```python
from build123d import *

# Parameters (mm, degrees)
F0_W        = 104.8084236681
F0_H        = 91.941319406
F1_DEPTH    = 3
F2_W        = 41.4473675191
F2_H        = 39.6052636206
F3_DEPTH    = 30
F4_T        = 3
F4_T3_DEPTH = 47.4473675191
F4_T5_DEPTH = 45.6052636206


# Not quite as in the source:
# - a shell that OpenCascade refuses in one call is made with other operations: the cavity is built on its own and cut out


with BuildPart() as f1:
    # F0 (on Top) → F1 (new body)
    with BuildSketch(Plane.XY):
        with Locations((0.5848687142, -2.3394748569)):
            Rectangle(F0_W, F0_H)
    extrude(amount=F1_DEPTH)

    # F2 (on face) → F3 (join)
    with BuildSketch(Plane.XY.offset(3)):
        with Locations((-0.575657934, -1.7269738019)):
            Rectangle(F2_W, F2_H)
    extrude(amount=F3_DEPTH)

    # F4: shell of thickness 3, made by hand


with BuildPart() as f4_core1:
    # F4_t2: copy of F1
    add(f1.part)

    # the walls: a layer under each face that stays
    f4_faces = [f4_core1.faces().sort_by_distance(p)[0] for p in [
        (0.5848687142, 43.6311848462, 1.5),
        (52.9890805483, -2.3394748569, 1.5),
        (-51.8193431199, -2.3394748569, 1.5),
        (-34.3512725085, -32.9865813255, 3),
        (0.5848687142, -48.3101345599, 1.5),
        (-0.575657934, 18.0756580085, 18),
        (-21.2993416935, -1.7269738019, 18),
        (-0.575657934, -21.5296056122, 18),
        (20.1480258256, -1.7269738019, 18),
        (-0.575657934, -1.7269738019, 33),
    ]]
    thicken(f4_faces, amount=-F4_T, mode=Mode.SUBTRACT)

    # F4_s4 → F4_t3 (cut)
    with BuildSketch(Plane.YZ.offset(-24.2993416935)):
        Polygon((18.1056580085, 3.03), (18.0756580085, 0), (15.0756580085, 0), (15.0756580085, 3), align=None)
        Polygon((-21.5596056122, 3.03), (-21.5296056122, 0), (-18.5296056122, 0), (-18.5296056122, 3), align=None)
    extrude(amount=F4_T3_DEPTH, mode=Mode.SUBTRACT)

    # F4_s6 → F4_t5 (cut)
    with BuildSketch(Plane.XZ.offset(-21.0756580085)):
        Polygon((-21.3293416935, 3.03), (-21.2993416935, 0), (-18.2993416935, 0), (-18.2993416935, 3), align=None)
        Polygon((20.1780258256, 3.03), (20.1480258256, 0), (17.1480258256, 0), (17.1480258256, 3), align=None)
    extrude(amount=F4_T5_DEPTH, mode=Mode.SUBTRACT)


with BuildPart() as f1_1:
    add(f1.part)

    # what is left inside the walls is the cavity
    f4_cavity = [f4_core1.part.solids().sort_by_distance(p)[0] for p in [
        (-0.575658, -7.327851, 0.03),
    ]]
    add(f4_cavity, mode=Mode.SUBTRACT)


solid = f1_1.part
```
Read the model definition and answer for the solid it produces. Units are mm, in the model's axes. A direction names the side the tool comes from. Coordinates: 2 decimals unless noted, no trailing zeros. Loops run counter-clockwise (first coordinate to the right, second up) from the corner with the lowest first, then second, coordinate; pieces in that order, holes last.
(1) The part is cut by section A-A (z = 14). Determine the outline of the cut face in (x, y).
Solution:
outline: (-21.3, -21.53) - (20.15, -21.53) - (20.15, 18.08) - (-21.3, 18.08) - close; hole (-18.3, -18.53) - (17.15, -18.53) - (17.15, 15.08) - (-18.3, 15.08) - close
(2) The part is cut by section D-D (x = -5). Determine the outline of the cut face in (y, z), and give its area (3 significant figures).
Solution:
outline: (-48.31, 0) - (-18.53, 0) - (-18.53, 30) - (15.08, 30) - (15.08, 0) - (43.63, 0) - (43.63, 3) - (18.08, 3) - (18.08, 33) - (-21.53, 33) - (-21.53, 3) - (-48.31, 3) - close
area: 456 mm2
(3) Flat-ended cylindrical pins translate along their axes: pin 1 Ø12 at (x, z) = (24, 17.5) entering from -Y; pin 2 Ø8 at (y, z) = (-26, 5.5) entering from -X; pin 3 Ø9 at (y, z) = (2, 16) entering from +X; pin 4 Ø4 at (x, z) = (-12, 5.5) entering from +Y. Find the tip coordinate at first contact, or state that the pin passes through.
Solution:
pin 1: stops at y = -21.53
pin 2: stops at x = -51.82
pin 3: stops at x = 20.15
pin 4: stops at y = 18.08
(4) The mould has two halves that part along Y. Classify faces 1 (the face through (-1, -21.53, 18)), 2 (the face through (17.148, -1, 15)), 3 (the face through (-21.299, -2, 18)): released by +Y, released by -Y, zero draft, split by the parting line, or undercut.
Solution:
face 1: released by -Y
face 2: undercut
face 3: zero draft
(5) A tool of negligible diameter and unlimited length cuts with its end or side. For faces 4 (the face through (-1, 18.076, 18)), 5 (the face through (52.989, -3, 1)), 6 (the face through (-1, -1, 30)), 7 (the face through (-1, -1, 33)), 8 (the face through (20.148, -2, 18)), from which of +Z, -Z, +X, -X, +Y, -Y can it reach the whole face along a straight path? Write none if from no direction.
Solution:
face 4: +Z, +X, -X, +Y
face 5: +Z, -Z, +X, +Y, -Y
face 6: -Z
face 7: +Z, +X, -X, +Y, -Y
face 8: +Z, +X, +Y, -Y
(6) Consider line 1 along X through (y, z) = (14.5, 19.5); line 2 along Y through (x, z) = (-18, 2.5); line 3 along Y through (x, z) = (13, 5). Determine where each line is inside the solid, lowest interval first.
Solution:
line 1: x = -21.3 to -18.3, 17.15 to 20.15
line 2: y = -48.31 to -18.53, 15.08 to 43.63
line 3: y = -21.53 to -18.53, 15.08 to 18.08
(7) The part is cut by section C-C (y = 5). Determine the outline of the cut face in (x, z), and give its area (3 significant figures).
Solution:
outline: (-51.82, 0) - (-18.3, 0) - (-18.3, 30) - (17.15, 30) - (17.15, 0) - (52.99, 0) - (52.99, 3) - (20.15, 3) - (20.15, 33) - (-21.3, 33) - (-21.3, 3) - (-51.82, 3) - close
area: 494 mm2
(8) The part is cut by section B-B (x = 18.5). Determine the outline of the cut face in (y, z).
Solution:
outline: (-48.31, 0) - (43.63, 0) - (43.63, 3) - (18.08, 3) - (18.08, 33) - (-21.53, 33) - (-21.53, 3) - (-48.31, 3) - close
